```python
from build123d import *

# Parameters (mm, degrees)
F0_R      = 22.5
F1_DEPTH  = 24
F2_DEPTH  = 21
F3_R      = 4
F4_DEPTH  = 7.8
F5_R      = 7.5
F6_DEPTH  = 3
F10_DEPTH = 9
F11_R     = 1
F12_R     = 27.8
F13_DEPTH = 22
F14_R     = 35
F15_DEPTH = 6.5
F16_R     = 3.5
F17_DEPTH = 3.8
F19_R     = 11
F20_DEPTH = 25
F22_R     = 11
F23_DEPTH = 25
F24_R     = 8.5
F25_DEPTH = 9
F26_R     = 12.5
F27_DEPTH = 23.5
F28_SIZE  = 2
F29_R     = 5.25
F30_DEPTH = 55
F31_R     = 8.25
F32_DEPTH = 9.5
F33_R     = 12.5
F36_SIZE  = 2
F37_R     = 9.0275939992
F38_DEPTH = 37
F39_R     = 4
F40_DEPTH = 15


with BuildPart() as f1:
    # F0 (on Front) → F1 (new body)
    with BuildSketch(Plane.XZ):
        Circle(F0_R)
    extrude(amount=F1_DEPTH)

    # F0 (on Front) → F2 (join)
    with BuildSketch(Plane.XZ):
        Circle(F0_R)
    extrude(amount=-F2_DEPTH)

    # F3 (on Front) → F4 (join)
    with BuildSketch(Plane.XZ):
        with BuildLine():
            Line((-9.3, 20.4880452948), (-40.3933333333, 6.3740585361))
            ThreePointArc((-40.3933333333, 6.3740585361), (-44.5, 0), (-40.3933333333, -6.3740585361))
            Line((-40.3933333333, -6.3740585361), (-9.3, -20.4880452948))
            ThreePointArc((-9.3, -20.4880452948), (-22.5, 0), (-9.3, 20.4880452948))
        make_face()
        with Locations((-37.5, 0)):
            Circle(F3_R, mode=Mode.SUBTRACT)
        with BuildLine():
            Line((9.3, -20.4880452948), (40.3933333333, -6.3740585361))
            ThreePointArc((40.3933333333, -6.3740585361), (44.5, 0), (40.3933333333, 6.3740585361))
            Line((40.3933333333, 6.3740585361), (9.3, 20.4880452948))
            ThreePointArc((9.3, 20.4880452948), (22.5, 0), (9.3, -20.4880452948))
        make_face()
        with Locations((37.5, 0)):
            Circle(F3_R, mode=Mode.SUBTRACT)
    extrude(amount=-F4_DEPTH)

    # F5 (on face) → F6 (join)
    with BuildSketch(Plane.XZ.offset(24)):
        Circle(F5_R)
    extrude(amount=F6_DEPTH)

    # F7 (on Top) → F8 (revolve)
    with BuildSketch(Plane.XY):
        Polygon((12.5, -27), (7.5, -27), (0, -27), (0, -38.8), (0, -41.7667143047), (12.5, -41.7667143047), (12.5, -38.8), (44.9961982667, -46), (49, -46), (49, -43), (35, -38.8), (35, -34.2), (49, -30), (49, -27), (44.9961982667, -27), (23.7909853458, -30), (12.5, -30), align=None)
    revolve(axis=Axis((0, -32.9, 0), (0, 1, 0)))

    # F9 (on face) → F10 (join)
    with BuildSketch(Plane.XZ.offset(41.7667143047)):
        Polygon((6.5, -3.7527767497), (6.5, 3.7527767497), (0, 7.5055534995), (-6.5, 3.7527767497), (-6.5, -3.7527767497), (0, -7.5055534995), align=None)
    extrude(amount=F10_DEPTH)

    # F11
    f11_edges = [f1.edges().sort_by_distance(p)[0] for p in [
        (6.5, -50.766714, 0),
        (3.25, -50.766714, 5.629165),
        (-3.25, -50.766714, 5.629165),
        (-6.5, -50.766714, 0),
        (-3.25, -50.766714, -5.629165),
        (3.25, -50.766714, -5.629165),
    ]]
    fillet(f11_edges, radius=F11_R)

    # F12 (on face) → F13 (join)
    with BuildSketch(Plane(origin=(0, 21, 0), x_dir=(-1, 0, 0), z_dir=(0, 1, 0))):
        Circle(F12_R)
    extrude(amount=F13_DEPTH)

    # F14 (on face) → F15 (join)
    with BuildSketch(Plane(origin=(0, 43, 0), x_dir=(-1, 0, 0), z_dir=(0, 1, 0))):
        Circle(F14_R)
    extrude(amount=F15_DEPTH)

    # F16 (on face) → F17 (join)
    with BuildSketch(Plane(origin=(0, 49.5, 0), x_dir=(-1, 0, 0), z_dir=(0, 1, 0))):
        with Locations((0, 30)):
            Circle(F16_R)
        Polygon((0, 32.3094010768), (2, 31.1547005384), (2, 28.8452994616), (0, 27.6905989232), (-2, 28.8452994616), (-2, 31.1547005384), align=None, mode=Mode.SUBTRACT)
        with Locations((-25.9807621135, 15)):
            Circle(F16_R)
        Polygon((-27.9807621135, 16.1547005384), (-25.9807621135, 17.3094010768), (-23.9807621135, 16.1547005384), (-23.9807621135, 13.8452994616), (-25.9807621135, 12.6905989232), (-27.9807621135, 13.8452994616), align=None, mode=Mode.SUBTRACT)
        with Locations((-25.9807621135, -15)):
            Circle(F16_R)
        Polygon((-27.9807621135, -16.1547005384), (-27.9807621135, -13.8452994616), (-25.9807621135, -12.6905989232), (-23.9807621135, -13.8452994616), (-23.9807621135, -16.1547005384), (-25.9807621135, -17.3094010768), align=None, mode=Mode.SUBTRACT)
        with Locations((0, -30)):
            Circle(F16_R)
        Polygon((0, -32.3094010768), (-2, -31.1547005384), (-2, -28.8452994616), (0, -27.6905989232), (2, -28.8452994616), (2, -31.1547005384), align=None, mode=Mode.SUBTRACT)
        with Locations((25.9807621135, -15)):
            Circle(F16_R)
        Polygon((27.9807621135, -16.1547005384), (25.9807621135, -17.3094010768), (23.9807621135, -16.1547005384), (23.9807621135, -13.8452994616), (25.9807621135, -12.6905989232), (27.9807621135, -13.8452994616), align=None, mode=Mode.SUBTRACT)
        with Locations((25.9807621135, 15)):
            Circle(F16_R)
        Polygon((27.9807621135, 16.1547005384), (27.9807621135, 13.8452994616), (25.9807621135, 12.6905989232), (23.9807621135, 13.8452994616), (23.9807621135, 16.1547005384), (25.9807621135, 17.3094010768), align=None, mode=Mode.SUBTRACT)
    extrude(amount=F17_DEPTH)

    # F19 (on offset) → F20 (join)
    with BuildSketch(Plane.YZ.offset(-40)):
        with Locations((37, 0)):
            Circle(F19_R)
    extrude(amount=F20_DEPTH)

    # F22 (on offset) → F23 (join)
    with BuildSketch(Plane.XY.offset(40)):
        with Locations((0, 37)):
            Circle(F22_R)
    extrude(amount=-F23_DEPTH)

    # F24 (on face) → F25 (join)
    with BuildSketch(Plane.XY.offset(40)):
        with Locations((0, 37)):
            Circle(F24_R)
    extrude(amount=F25_DEPTH)

    # F26 (on face) → F27 (join)
    with BuildSketch(Plane.XY.offset(49)):
        with Locations((0, 37)):
            Circle(F26_R)
    extrude(amount=F27_DEPTH)

    # F28
    f28_edges = [f1.edges().sort_by_distance(p)[0] for p in [
        (-12.5, 37, 72.5),
    ]]
    chamfer(f28_edges, length=F28_SIZE)

    # F29 (on face) → F30 (cut)
    with BuildSketch(Plane.XY.offset(72.5)):
        with Locations((0, 37)):
            Circle(F29_R)
    extrude(amount=-F30_DEPTH, mode=Mode.SUBTRACT)

    # F31 (on face) → F32 (join)
    with BuildSketch(Plane(origin=(-40, 0, 0), x_dir=(0, -1, 0), z_dir=(-1, 0, 0))):
        with Locations((-37, 0)):
            Circle(F31_R)
    extrude(amount=F32_DEPTH)

    # F35: sweep along a path in F34
    with BuildLine(Plane.XY) as f35_path:
        Line((-49.5, 37), (-54.5, 37))
        ThreePointArc((-54.5, 37), (-75.7132034356, 45.7867965644), (-84.5, 67))
        Line((-84.5, 67), (-84.5, 106))
    # F33 (on face) → F35 (sweep)
    with BuildSketch(Plane(origin=(-49.5, 0, 0), x_dir=(0, -1, 0), z_dir=(-1, 0, 0))):
        with Locations((-37, 0)):
            Circle(F33_R)
    sweep(path=f35_path.line)

    # F36
    f36_edges = [f1.edges().sort_by_distance(p)[0] for p in [
        (-72, 106, 0),
    ]]
    chamfer(f36_edges, length=F36_SIZE)

    # F37 (on face) → F38 (cut)
    with BuildSketch(Plane(origin=(0, 106, 0), x_dir=(-1, 0, 0), z_dir=(0, 1, 0))):
        with Locations((84.5, 0)):
            Circle(F37_R)
    extrude(amount=-F38_DEPTH, mode=Mode.SUBTRACT)

    # F39 (on face) → F40 (join)
    with BuildSketch(Plane(origin=(0, 7.8, 0), x_dir=(-1, 0, 0), z_dir=(0, 1, 0))):
        with Locations((-37.5, 0)):
            Circle(F39_R)
        with Locations((37.5, 0)):
            Circle(F39_R)
    extrude(amount=-F40_DEPTH)


solid = f1.part
```
CAD build for the part. Positions are in the model's coordinates, mm. A direction names the side the tool comes from. Give positions to 0.01 mm unless a question says otherwise; leave off trailing zeros. Write each loop counter-clockwise with the first axis right and the second up, starting at its lowest first coordinate (ties: lowest second). Pieces come first, ordered by that corner, then holes. Notation, with made-up numbers: (86.5, 86) -> (94.5, 86) arc R32 ccw to (94.5, 115) -> close; hole circle Ø3 at (42.25, 86). An arc over 180 degrees is marked (long way). Write each question's results on one line, items separated by ' | '.
1. Wall check: probe 1 along Y at (x, z) = (1, 38); probe 2 along Y at (x, z) = (28.5, 4); probe 3 along Z at (x, y) = (-84, 84). Give the ranges that are in metal, low to high. Write a range as [from, to].
Geometry check:
probe 1: [-44.45, -39.7], [-33.3, -27.99], [26.05, 31.85], [42.15, 47.95] | probe 2: [-42.41, -29.29], [0, 7.8], [43, 49.5] | probe 3: [-12.49, -9.01], [9.01, 12.49]
2. Cut at B-B, the plane z = 58.5. Write the cut outline in (x, y), then the cut area to 3 significant figures.
Geometry check:
outline: circle Ø25 at (0, 37); hole circle Ø10.5 at (0, 37) | area: 404 mm²
3. Cut at D-D, the plane x = 37.5. Give the number of separate pieces and of enclosed holes in the cut face, then the cut area to 3 significant figures.
Geometry check:
separate pieces: 3 | enclosed holes: 0 | area: 750 mm²
4. Cut at A-A, the plane y = 88.5. Write the cut outline in (x, z), then the cut area to 3 significant figures.
Geometry check:
outline: circle Ø25 at (-84.5, 0); hole circle Ø18.06 at (-84.5, 0) | area: 235 mm²
5. Which spindle directions (+Z, -Z, +X, -X, +Y, -Y) get a long thin tool onto all of the face, cutting with end or side? Do faces 4 (the cylindrical face through (26.739, 51.373, 11.583)), 5 (the flat face through (0, -24, -10)), 6 (the cylindrical face through (-2.71, 24.797, 59.6)). Say none if no direction does.
Geometry check:
face 4: +Y | face 5: none | face 6: +Z
6. Cut at C-C, the plane y = 11. Write the cut outline in (x, z), then the cut area to 3 significant figures.
Geometry check:
outline: circle Ø45 at (0, 0) | area: 1,590 mm²
7. Drop flat-ended pins along their axis: P1, Ø10.5, axis at x = -22, z = -4, coming from the -Y side; P2, Ø4.5, axis at x = -0.5, z = -30.5, coming from the +Y side; P3, Ø8, axis at x = 26, z = 26.5, coming from the +Y side. Give the stop position or say it passes through.
Geometry check:
P1: y = -42.15 | P2: y = 53.3 | P3: y = 49.5
8. Two-plate mould, pull along Z, no slides. Class faces 1 (the flat face through (0, 49.5, 30)), 2 (the flat face through (28, 0, -1)), 3 (the cylindrical face through (-52.035, 46.92, -7.606)): pulls with the +Z half, pulls with the -Z half, needs draft (parallel to the pull), parting line crosses it, or undercut.
Geometry check:
face 1: undercut | face 2: needs draft | face 3: parting line crosses it
